from build123d import *

# Parameters (mm, degrees)
SKETCH1_W                      = 95
SKETCH1_H                      = 95
BOSS_EXTRUDE1_DEPTH            = 1
EDGE_FLANGE1_STRIP_W           = 6
EDGE_FLANGE1_STRIP_H           = 1
EDGE_FLANGE1_STRIP_CUT_DEPTH   = 95
EDGE_FLANGE1_STRIP_2_W         = 6
EDGE_FLANGE1_STRIP_2_H         = 1
EDGE_FLANGE1_STRIP_CUT_2_DEPTH = 95
EDGE_FLANGE1_DEPTH             = 95
EDGE_FLANGE1_BEND_DEPTH        = 95


# Sheet-metal steps are written as plain solids
with BuildPart() as part:
    # Sketch1 → Boss-Extrude1 (new body)
    with BuildSketch(Plane(origin=(0, 0, 0), x_dir=(1, 0, 0), z_dir=(0, 1, 0))):
        Rectangle(SKETCH1_W, SKETCH1_H)
    extrude(amount=BOSS_EXTRUDE1_DEPTH)

    # Edge-Flange1 strip (across the edge) → Edge-Flange1 strip cut (cut)
    with BuildSketch(Plane(origin=(-47.5, 1, -47.5), x_dir=(1, 0, 0), z_dir=(0, 0, 1))):
        with Locations((-1, -0.5)):
            Rectangle(EDGE_FLANGE1_STRIP_W, EDGE_FLANGE1_STRIP_H)
    extrude(amount=EDGE_FLANGE1_STRIP_CUT_DEPTH, mode=Mode.SUBTRACT)

    # Edge-Flange1 strip 2 (across the edge) → Edge-Flange1 strip cut 2 (cut)
    with BuildSketch(Plane(origin=(47.5, 1, 47.5), x_dir=(-1, 0, 0), z_dir=(0, 0, -1))):
        with Locations((-1, -0.5)):
            Rectangle(EDGE_FLANGE1_STRIP_2_W, EDGE_FLANGE1_STRIP_2_H)
    extrude(amount=EDGE_FLANGE1_STRIP_CUT_2_DEPTH, mode=Mode.SUBTRACT)

    # Edge-Flange1 section (across the edge) → Edge-Flange1 (add)
    with BuildSketch(Plane(origin=(-47.5, 1, -47.5), x_dir=(1, 0, 0), z_dir=(0, 0, 1))):
        with BuildLine():
            Line((0, 1), (0, 19))
            Line((0, 19), (1, 19))
            Line((1, 19), (1, 1))
            ThreePointArc((1, 1), (1.292893219, 0.292893219), (2, 0))
            Line((2, 0), (2, -1))
            ThreePointArc((2, -1), (0.585786438, -0.414213562), (0, 1))
        make_face()
    extrude(amount=EDGE_FLANGE1_DEPTH)

    # Edge-Flange1 section 2 (across the edge) → Edge-Flange1 bend (add)
    with BuildSketch(Plane(origin=(47.5, 1, 47.5), x_dir=(-1, 0, 0), z_dir=(0, 0, -1))):
        with BuildLine():
            Line((0, 1), (0, 19))
            Line((0, 19), (1, 19))
            Line((1, 19), (1, 1))
            ThreePointArc((1, 1), (1.292893219, 0.292893219), (2, 0))
            Line((2, 0), (2, -1))
            ThreePointArc((2, -1), (0.585786438, -0.414213562), (0, 1))
        make_face()
    extrude(amount=EDGE_FLANGE1_BEND_DEPTH)


solid = part.part
For this review, take the finished solid that the model builds, in its own axes (mm). A direction names the side the tool comes from. Round coordinates to 2 decimals unless told otherwise and drop trailing zeros. Loops run counter-clockwise (first coordinate to the right, second up) from the corner with the lowest first, then second, coordinate; pieces in that order, holes last. Notation, with made-up numbers: (79, 82) - (126, 82) arc R11 cw to (126, 98) - close; hole circle Ø8 at (61.25, 40.25). An arc over 180 degrees is marked (long way). One line per question, with ' | ' between items.
Q1. The part is to be moulded in two halves that separate along X. For faces 3 (the flat face through (46.5, 11, 1)), 4 (the flat face through (47.5, 11, 1)), 5 (the flat face through (-46.5, 11, -1)), 6 (the flat face through (-1, 0, -1)), say which applies: released by +X, released by -X, zero draft, split by the parting line, or undercut.
Taken from the geometry:
face 3: undercut | face 4: released by +X | face 5: undercut | face 6: zero draft
Q2. Take a section at C-C (x = 36.5). Give the boundary of the cut face in (y, z), and give its area (3 significant figures).
Taken from the geometry:
outline: (0, -47.5) - (1, -47.5) - (1, 47.5) - (0, 47.5) - close | area: 95.0 mm²
Q3. For pin 1 (8 mm diameter, centred on x = 20.5, y = 4.5, fed in from -Z), flat-tipped, find the tip position at first contact; note if it passes through.
Taken from the geometry:
pin 1: stops at z = -47.5
Q4. For line 1 along X through (y, z) = (4.5, -34.5); line 2 along Y through (x, z) = (-35, 42), list the stretches that pass through material, from the lowest coordinate up. Write a range as [from, to].
Taken from the geometry:
line 1: x = [-47.5, -46.5], [46.5, 47.5] | line 2: y = [0, 1]
Q5. Take a section at A-A (y = 10.25). Give the boundary of the cut face in (x, z).
Taken from the geometry:
outline: (-47.5, -47.5) - (-46.5, -47.5) - (-46.5, 47.5) - (-47.5, 47.5) - close; (46.5, -47.5) - (47.5, -47.5) - (47.5, 47.5) - (46.5, 47.5) - close
Q6. Tool access review of faces 1 (the flat face through (-47.5, 11, -1)), 2 (the flat face through (-1, 1, -1)): name each direction out of +Z, -Z, +X, -X, +Y, -Y from which nothing blocks a thin tool from reaching the whole face with its end or side.
Taken from the geometry:
face 1: +Z, -Z, -X, +Y, -Y | face 2: +Z, -Z, +Y
Q7. Take a section at B-B (z = 9). Give the boundary of the cut face in (x, y).
Taken from the geometry:
outline: (-47.5, 2) arc R2 ccw to (-45.5, 0) - (45.5, 0) arc R2 ccw to (47.5, 2) - (47.5, 20) - (46.5, 20) - (46.5, 2) arc R1 cw to (45.5, 1) - (-45.5, 1) arc R1 cw to (-46.5, 2) - (-46.5, 20) - (-47.5, 20) - close
